Here's how the part is built. I have some questions about the finished solid (model axes, mm). A direction names the side the tool comes from. Round coordinates to 2 decimals unless told otherwise and drop trailing zeros. Order: outer loops, then holes, each group sorted by start corner. A loop starts at its lowest first (then second) coordinate and runs counter-clockwise, first axis right, second up.
```python
from build123d import *

# Parameters (mm, degrees)
SKETCH1_R           = 75
BOSS_EXTRUDE3_DEPTH = 19.2
SKETCH3_R           = 70
CUT_EXTRUDE1_DEPTH  = 9.6
SKETCH4_R           = 30
BOSS_EXTRUDE4_DEPTH = 30
SKETCH5_R           = 10
CUT_EXTRUDE2_DEPTH  = 57
SKETCH6_R           = 4
CUT_EXTRUDE3_DEPTH  = 57
SKETCH7_W           = 6
SKETCH7_H           = 6
CUT_EXTRUDE4_DEPTH  = 114.217313164


with BuildPart() as part:
    # Sketch1 → Boss-Extrude3 (new body)
    with BuildSketch(Plane.XY):
        Circle(SKETCH1_R)
    extrude(amount=BOSS_EXTRUDE3_DEPTH)

    # Sketch3 → Cut-Extrude1 (cut)
    with BuildSketch(Plane.XY.offset(19.2)):
        Circle(SKETCH3_R)
    extrude(amount=-CUT_EXTRUDE1_DEPTH, mode=Mode.SUBTRACT)

    # Sketch4 → Boss-Extrude4 (add)
    with BuildSketch(Plane.XY.offset(9.6)):
        Circle(SKETCH4_R)
    extrude(amount=BOSS_EXTRUDE4_DEPTH)

    # Sketch5 → Cut-Extrude2 (cut)
    with BuildSketch(Plane.XY.offset(39.6)):
        Circle(SKETCH5_R)
    extrude(amount=-CUT_EXTRUDE2_DEPTH, mode=Mode.SUBTRACT)

    # Sketch6 → Cut-Extrude3 (cut)
    with BuildSketch(Plane.XY.offset(9.6)):
        with Locations((0, 60)):
            Circle(SKETCH6_R)
        with Locations((60, 0)):
            Circle(SKETCH6_R)
        with Locations((0, -60)):
            Circle(SKETCH6_R)
        with Locations((-60, 0)):
            Circle(SKETCH6_R)
    extrude(amount=-CUT_EXTRUDE3_DEPTH, mode=Mode.SUBTRACT)

    # Sketch7 → Cut-Extrude4 (cut, through all)
    with BuildSketch(Plane.XY.offset(39.6)):
        with Locations((0, 10)):
            Rectangle(SKETCH7_W, SKETCH7_H)
    extrude(amount=-CUT_EXTRUDE4_DEPTH, mode=Mode.SUBTRACT)


solid = part.part
```
1. If we section it at C-C, the plane x = -60: Write out the boundary of the cut face in (y, z), and give its area (3 significant figures).
Evaluation:
outline: (-45, 0) - (-4, 0) - (-4, 9.6) - (-36.06, 9.6) - (-36.06, 19.2) - (-45, 19.2) - close; (4, 0) - (45, 0) - (45, 19.2) - (36.06, 19.2) - (36.06, 9.6) - (4, 9.6) - close
area: 959 mm2
2. I'm going to push flat-ended pins straight in: P1, Ø1.5, axis at x = -46, y = -50, coming from the -Z side; P2, Ø4, axis at y = 12, z = 11.5, coming from the +X side; P3, Ø5, axis at y = -20, z = 31, coming from the +X side; P4, Ø13, axis at x = -60, y = 0, coming from the +Z side. Where does each tip first touch, or does it pass through?
Evaluation:
P1: stops at z = 0
P2: stops at x = 74.33
P3: stops at x = 24.37
P4: stops at z = 9.6
3. If we section it at A-A, the plane z = 5: Write out the boundary of the cut face in (x, y).
Evaluation:
outline: circle Ø150 at (0, 0); hole circle Ø8 at (-60, 0); hole circle Ø8 at (0, -60); hole circle Ø8 at (0, 60); hole (-3, 9.54) arc R10 ccw (long way) to (3, 9.54) - (3, 13) - (-3, 13) - close; hole circle Ø8 at (60, 0)
4. If we section it at B-B, the plane y = 0: Write out the boundary of the cut face in (x, z), and give its area (3 significant figures).
Evaluation:
outline: (-75, 0) - (-64, 0) - (-64, 9.6) - (-70, 9.6) - (-70, 19.2) - (-75, 19.2) - close; (-56, 0) - (-10, 0) - (-10, 39.6) - (-30, 39.6) - (-30, 9.6) - (-56, 9.6) - close; (10, 0) - (56, 0) - (56, 9.6) - (30, 9.6) - (30, 39.6) - (10, 39.6) - close; (64, 0) - (75, 0) - (75, 19.2) - (70, 19.2) - (70, 9.6) - (64, 9.6) - close
area: 2,390 mm2
5. If we mould it in two halves opening along X, with no side actions, what happens to faces 4 (the cylindrical face through (-29.97, 1.32, 24.39)), 5 (the flat face through (13, 0, 39.6)), 6 (the cylindrical face through (63.815, 1.201, 4.867)), 7 (the cylindrical face through (-9.764, 74.362, 9.466))? For each: released by +X, released by -X, zero draft, split by the parting line, or undercut.
Evaluation:
face 4: undercut
face 5: zero draft
face 6: undercut
face 7: split by the parting line
6. On a 3-axis mill with a long thin cutter (end or side, diameter ignored), from which of +Z, -Z, +X, -X, +Y, -Y can I reach the whole of each face in a straight line? I mean faces 1 (the flat face through (-3, 11, 20)), 2 (the flat face through (50, -50, 19.2)), 3 (the flat face through (16, 1, 0)). Say none if no direction works.
Evaluation:
face 1: +Z, -Z
face 2: +Z
face 3: -Z, +X, -X, +Y, -Y
7. I need wall thicknesses on probe 1 along Y at (x, z) = (0, 15); probe 2 along Y at (x, z) = (0, 4); probe 3 along Z at (x, y) = (-56.5, -17.5). Which ranges of each line are inside material? Lowest first, please.
Evaluation:
probe 1: y = -75 to -70, -30 to -10, 13 to 30, 70 to 75
probe 2: y = -75 to -64, -56 to -10, 13 to 56, 64 to 75
probe 3: z = 0 to 9.6
